from build123d import *

# Parameters (mm, degrees)
SKETCH1_R           = 9.1
SKETCH1_R_2         = 6.1
BOSS_EXTRUDE1_DEPTH = 10
SKETCH2_R           = 9.1
SKETCH2_R_2         = 3.1
BOSS_EXTRUDE2_DEPTH = 3
BOSS_EXTRUDE3_DEPTH = 3


with BuildPart() as part:
    # Sketch1 → Boss-Extrude1 (new body)
    with BuildSketch(Plane(origin=(0, 0, 0), x_dir=(1, 0, 0), z_dir=(0, 1, 0))):
        with Locations(Location((0, 0, 0), (0, 0, 270))):
            Circle(SKETCH1_R)
        with Locations(Location((0, 0, 0), (0, 0, 270))):
            Circle(SKETCH1_R_2, mode=Mode.SUBTRACT)
    extrude(amount=BOSS_EXTRUDE1_DEPTH)

    # Sketch2 → Boss-Extrude2 (add)
    with BuildSketch(Plane(origin=(0, 10, 0), x_dir=(1, 0, 0), z_dir=(0, 1, 0))):
        with Locations(Location((0, 0, 0), (0, 0, 270))):
            Circle(SKETCH2_R)
        with Locations(Location((0, 0, 0), (0, 0, 270))):
            Circle(SKETCH2_R_2, mode=Mode.SUBTRACT)
    extrude(amount=BOSS_EXTRUDE2_DEPTH)

    # Sketch3 → Boss-Extrude3 (add)
    with BuildSketch(Plane(origin=(0, 13, 0), x_dir=(1, 0, 0), z_dir=(0, 1, 0))):
        Polygon((-9.1, 0), (-24.1, 0), (-24.1, -20.018492189), (24.1, -20.018492189), (24.1, 0), (9.1, 0), (0, -6.029666322), align=None)
    extrude(amount=-BOSS_EXTRUDE3_DEPTH)


solid = part.part
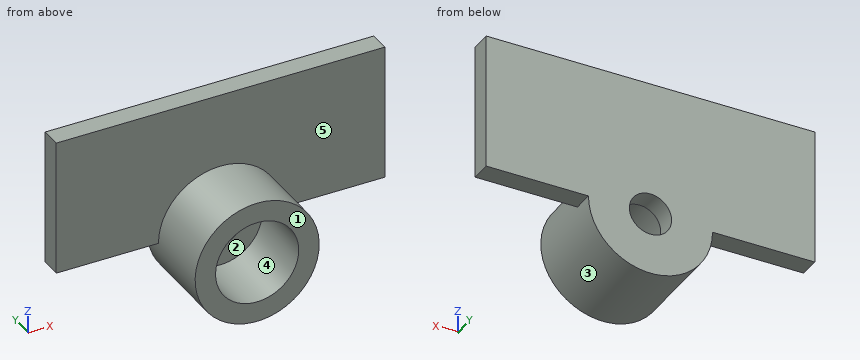
Input: part model. Units: mm. Frame: model coordinates. Face numbers are marked on the shaded views. A direction names the side the tool comes from. Coordinates: 2 decimals unless noted, no trailing zeros. Loops run counter-clockwise (first coordinate to the right, second up) from the corner with the lowest first, then second, coordinate; pieces in that order, holes last.
Q1. Cut plane A-A (y = 10.5). Output: boundary loops of the cut face in (x, z).
Q2. Draft query along Z for the marked faces 3, 4 and 5. Return one class per face: +Z half, -Z half, draft (parallel to the pull), parting line (faces both ways), or undercut.
Q3. Set-up query: the marked faces 1 and 2. Return all of +Z, -Z, +X, -X, +Y, -Y with unobstructed straight access to the full face (end or side cutting, diameter ignored); none if empty.
Q4. Material intervals for line 1 (X direction, y = 4, z = 0); line 2 (Y direction, x = -5, z = 16.5); line 3 (Z direction, x = -2.5, y = 9.5), sorted ascending.
Q5. Cut plane D-D (x = -11.5). Output: boundary loops of the cut face in (y, z), then the cut area to 3 significant figures.
Q6. Cut plane B-B (x = 0). Output: boundary loops of the cut face in (y, z), then the cut area to 3 significant figures.
Q7. Cut plane C-C (z = 16.25). Output: boundary loops of the cut face in (x, y).
Q8. Contact query for flat-ended pins moving along their axis: pin 1 (3.5 mm diameter, centred on x = -18, y = 12, fed in from -Z); pin 2 (5.5 mm diameter, centred on x = 0, z = 0, fed in from +Y); pin 3 (11 mm diameter, centred on x = 0, z = 0, fed in from -Y). Output: stop coordinate, or through.
Working result:
1. outline: (-24.1, 0) - (-9.1, 0) arc R9.1 ccw to (9.1, 0) - (24.1, 0) - (24.1, 20.02) - (-24.1, 20.02) - close; hole circle Ø6.2 at (0, 0)
2. face 3: parting line
2. face 4: undercut
2. face 5: draft
3. face 1: +Z, -Z, +X, -X, -Y
3. face 2: -Y
4. line 1: x = -9.1 to -6.1, 6.1 to 9.1
4. line 2: y = 10 to 13
4. line 3: z = -8.75 to -5.56, 5.56 to 8.75
5. outline: (10, 0) - (13, 0) - (13, 20.02) - (10, 20.02) - close
5. area: 60.1 mm2
6. outline: (0, -9.1) - (13, -9.1) - (13, -3.1) - (10, -3.1) - (10, -6.1) - (0, -6.1) - close; (0, 6.1) - (10, 6.1) - (10, 3.1) - (13, 3.1) - (13, 20.02) - (10, 20.02) - (10, 9.1) - (0, 9.1) - close
6. area: 129 mm2
7. outline: (-24.1, 10) - (24.1, 10) - (24.1, 13) - (-24.1, 13) - close
8. pin 1: stops at z = 0
8. pin 2: passes through
8. pin 3: stops at y = 10
